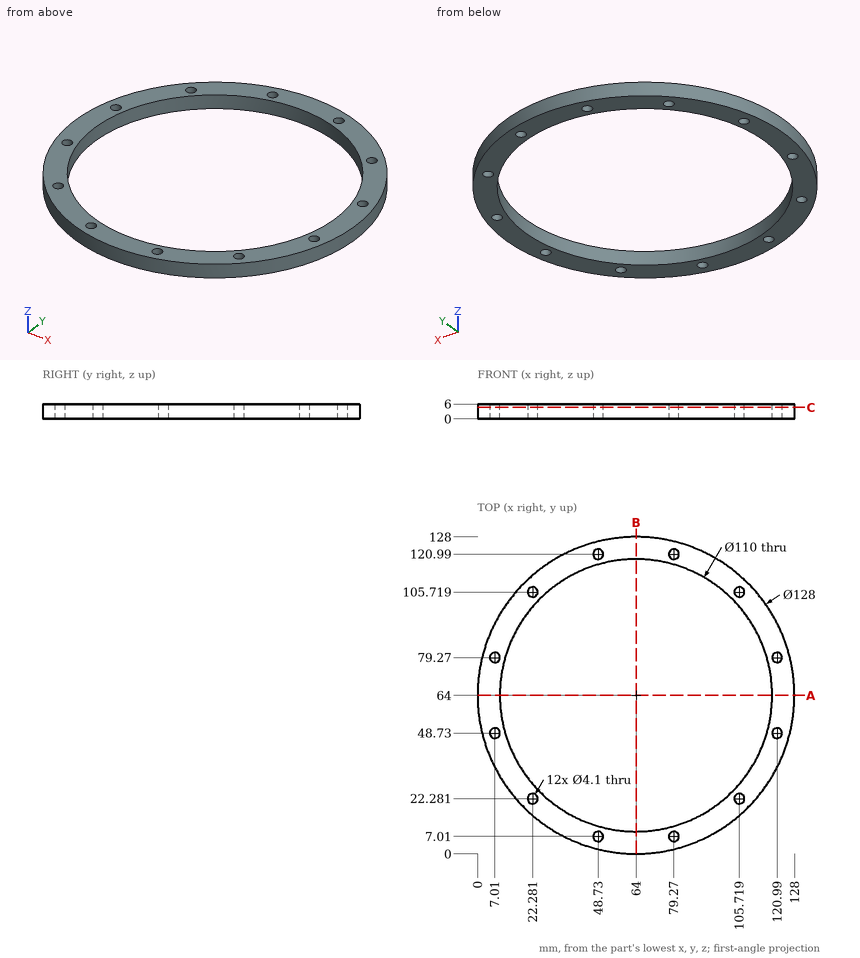
Job drawing, mm, ordinate dimensions from the low corner. One solid piece. Give positions to 0.01 mm unless a question says otherwise; leave off trailing zeros. Loops run counter-clockwise (first coordinate to the right, second up) from the corner with the lowest first, then second, coordinate; pieces in that order, holes last. Notation, with made-up numbers: (-37, 59.25) -> (7, 59.25) arc R9 ccw to (7, 75.25) -> close; hole circle Ø3 at (6.25, 32.25). An arc over 180 degrees is marked (long way). Use a Markdown table: item, result. Add a question column.
(1) Slice it at C-C on z = 4.65. Give the number of separate pieces and of enclosed holes in the cut face, and give its area (3 significant figures).
(2) Slice it at A-A on y = 64. List the corners of the cut face in (x, z).
(3) Wall check: line 1 along Y through (x, z) = (8.5, 3.8) (1 decimal); line 2 along X through (y, z) = (48, 0.7) (1 decimal); line 3 along Y through (x, z) = (105.5, 4.4) (1 decimal). Give the ranges that are in metal, low to high.
(4) Drop flat-ended pins along their axis: pin 1 Ø3.5 at (x, y) = (48.73, 120.99) entering from +Z; pin 2 Ø3 at (y, z) = (26, 2.5) entering from -X. Give the stop position or say it passes through.
Filled sheet:
| question | item | result |
|---|---|---|
| 1 | separate pieces | 1 |
| 1 | enclosed holes | 13 |
| 1 | area | 3,210 mm2 |
| 2 | outline | (0, 0) -> (9, 0) -> (9, 6) -> (0, 6) -> close; (119, 0) -> (128, 0) -> (128, 6) -> (119, 6) -> close |
| 3 | line 1 | 32.1 to 47.3, 50.1 to 77.9, 80.7 to 95.9 |
| 3 | line 2 | 2 to 5.1, 8.9 to 11.4, 116.6 to 119.1, 122.9 to 126 |
| 3 | line 3 | 15.3 to 20.2, 24.3 to 27.9, 100.1 to 103.7, 107.8 to 112.7 |
| 4 | pin 1 | through |
| 4 | pin 2 | x = 11.43 |
